Autodesk Inventor part; units mm, degrees
ref_plane "Work Plane1" through (22.5184, 2.463, -18.3509) normal (0, 0, 1) x (0.9997722, -0.0213418, 0)
ref_plane "YZ Plane" through (0, 0, 0) normal (1, 0, 0) x (0, 1, 0)
ref_plane "XZ Plane" through (0, 0, 0) normal (0, 1, 0) x (-1, 0, 0)
ref_plane "Work Plane1" through (22.5184, 2.463, -18.3509) normal (0, 0, 1) x (0.9997722, -0.0213418, 0)
sketch "ThermoBulbBorder" plane through (22.5184, 2.463, -18.3509) normal (0, 0, 1) x (0.9997722, -0.0213418, 0)
  arc A0 (-447.455, -468.958) -> (162.145, -468.958) centre (-142.655, -774.8145) ccw
  arc A1 (-447.455, -468.958) -> (162.145, -468.958) centre (-142.655, -774.8145) ccw
  arc A2 (-383.955, -588.5959) -> (98.645, -588.5959) centre (-142.655, -774.8145) ccw
  line L0 (-447.455, -468.958) -> (-383.955, -468.958)
  line L1 (-383.955, -468.958) -> (-383.955, -588.5959)
  line L2 (162.145, -468.958) -> (98.645, -468.958)
  line L3 (98.645, -468.958) -> (98.645, -588.5959)
  line L4 (-383.955, -961.033) -> (-484.4967, -1038.6241)
  line L5 (98.645, -961.033) -> (199.1867, -1038.6241)
  arc A3 (-447.455, -468.958) -> (162.145, -468.958) centre (-142.655, -774.8145) ccw
  circle A4 centre (-142.655, -774.8145) radius 419.1 construction
  circle A5 centre (-142.655, -774.8145) radius 410.972 construction
  circle A6 centre (-142.655, -774.8145) radius 353.822 construction
  circle A7 centre (-142.655, -774.8145) radius 345.694 construction
  line L6 (98.645, -468.958) -> (98.645, -316.558) construction
  line L7 (-383.955, -468.958) -> (-383.955, -316.558) construction
  dimension "d0" = 609.6
  dimension "d5" = 63.5
  dimension "d6" = 63.5
  dimension "d7" = 838.2
  dimension "d8" = 8.128
  dimension "d9" = 8.128
  dimension "d10" = 57.15
  dimension "d11" = 40.894
  dimension "d12" = 152.4
extrude "Extrusion3" add sketch "ThermoBulbBorder" along normal blind 18.034 contours L5 A2 L3 L2 A0
sketch "Sketch2" plane through (22.5184, 2.463, -0.3169) normal (0, 0, 1) x (0.9997722, -0.0213418, 0)
  line L0 (149.445, -468.958) -> (137.253, -468.958)
  arc A0 (199.1867, -1038.6241) -> (162.145, -468.958) centre (-142.655, -774.8145) ccw
  arc A1 (124.5847, -981.0515) -> (98.645, -538.7528) centre (-142.655, -774.8145) ccw
  arc A2 (134.2367, -988.5003) -> (98.645, -521.6249) centre (-142.655, -774.8145) ccw
  arc A3 (179.4805, -1023.4163) -> (144.5742, -486.5897) centre (-142.655, -774.8145) ccw
  arc A4 (189.1325, -1030.865) -> (153.1803, -477.9538) centre (-142.655, -774.8145) ccw
  line L1 (162.145, -468.958) -> (98.645, -468.958)
  line L2 (98.645, -961.033) -> (199.1867, -1038.6241)
  line L3 (98.645, -538.7528) -> (98.645, -521.6249)
  line L4 (98.645, -468.958) -> (98.645, -588.5959)
  line L5 (124.5847, -981.0515) -> (134.2367, -988.5003)
  line L6 (179.4805, -1023.4163) -> (189.1325, -1030.865)
  line L7 (149.445, -468.958) -> (149.445, -443.558) construction
  arc A5 (149.445, -468.958) -> (153.1803, -477.9538) centre (162.145, -468.958) ccw
  line L8 (137.253, -468.958) -> (137.253, -443.558) construction
  arc A6 (137.253, -468.958) -> (144.5742, -486.5897) centre (162.145, -468.958) ccw
  point P0 (-22.4607, -2.943)
  dimension "d17" = 12.7
  dimension "bRopeChannel" = 12.192
  dimension "d19" = 12.192
  dimension "d20" = 57.15
  dimension "d23" = 12.7
  dimension "d24" = 25.4
  dimension "d25" = 12.192
extrude "Extrusion4" cut sketch "Sketch2" against normal blind 12.7 contours A5 A4 L2 A3 A6 L0 | A2 L2 A1 L3
equation "\"d6\" = d5"
equation "\"d8\" = sRopeChannel"
equation "\"d9\" = sRopeChannel"
equation "\"d19\" = bRopeChannel"
equation "\"d23\" = d17"
equation "\"sRopeChannel\" = 8.128"
properties part number "HOT Thermo bulb outline R" material "Rubber, Butyl"
Geometry: final body of the model. Coordinates: model frame, mm. A direction names the side the tool comes from. Round coordinates to 2 decimals unless told otherwise and drop trailing zeros. Write each loop counter-clockwise with the first axis right and the second up, starting at its lowest first coordinate (ties: lowest second). Pieces come first, ordered by that corner, then holes.
Item 1: Section query D-D (x = 251). Return loops of the section in (y, z).
Item 2: Mould query, pull axis X, two halves, no side actions, for faces 3 (the face through (200.8, -759.9, -6.6)), 4 (the face through (168.138, -772.831, -9.46)), 5 (the face through (287, -756, -0.317)). Classes: +X half, -X half, draft (parallel to the pull), parting line (faces both ways), or undercut.
Item 3: Pin query (flat end, axial travel): P1, Ø1.5, axis at x = 204, z = -3.5, coming from the +Y side. Return the tip coordinate at first contact, or that it passes through.
Item 4: Section query A-A (z = -9). Return loops of the section in (x, y), plus the area to 3 significant figures.
Item 5: Section query B-B (y = -624). Return loops of the section in (x, z).
Item 6: Set-up query: faces 1 (the face through (294.538, -745.954, -9.46)), 2 (the face through (212.772, -753.58, -6.578)). Return all of +Z, -Z, +X, -X, +Y, -Y with unobstructed straight access to the full face (end or side cutting, diameter ignored); none if empty.
Item 7: Material intervals for L1, parallel to Y at x = 227.5, z = -11.5; L2, parallel to X at y = -904, z = -2.25; L3, parallel to X at y = -892.5, z = -3.75, sorted ascending.
Item 8: Section query C-C (x = 119.5). Return loops of the section in (y, z).
Completed:
1. outline: (-959.36, -18.35) - (-578.9, -18.35) - (-578.9, -0.32) - (-609.82, -0.32) - (-609.82, -13.02) - (-645.4, -13.02) - (-645.4, -0.32) - (-892.86, -0.32) - (-892.86, -13.02) - (-928.44, -13.02) - (-928.44, -0.32) - (-959.36, -0.32) - close
2. face 3: undercut
2. face 4: -X half
2. face 5: draft
3. P1: stops at y = -502.81
4. outline: (100.63, -960.46) - (126.14, -981.02) arc R337.57 ccw to (109.64, -538.27) - (108.58, -588.1) arc R304.8 cw to start; (110.01, -521.15) arc R349.76 cw to (135.63, -988.68) - (180.12, -1024.55) arc R406.91 ccw to (156.67, -487.1) arc R24.89 cw to (149.73, -469.32) - (111.13, -468.49) - close; (161.92, -469.58) arc R12.7 ccw to (165.46, -478.65) arc R419.1 cw to (189.61, -1032.2) - (199.49, -1040.18) arc R431.8 ccw to (174.62, -469.85) - close
4. area: 55,300 mm2
5. outline: (131.39, -18.35) - (270.04, -18.35) - (270.04, -0.32) - (256.53, -0.32) - (256.53, -13.02) - (243.51, -13.02) - (243.51, -0.32) - (181.59, -0.32) - (181.59, -13.02) - (168.14, -13.02) - (168.14, -0.32) - (131.39, -0.32) - close
6. face 1: +Z, -Z, +X
6. face 2: +Z
7. L1: y = -1001.19 to -976.61, -950.72 to -587.54, -561.65 to -537.07
7. L2: x = 136.7 to 172.81, 186.07 to 247.27, 260.17 to 273.56
7. L3: x = 142.08 to 177.57, 190.64 to 251.12, 263.89 to 277.16
8. outline: (-975.67, -18.35) - (-934.34, -18.35) - (-934.34, -0.32) - (-975.67, -0.32) - close; (-603.92, -18.35) - (-468.67, -18.35) - (-468.67, -0.32) - (-530.96, -0.32) - (-530.96, -13.02) - (-549.26, -13.02) - (-549.26, -0.32) - (-603.92, -0.32) - close
